Read the model definition and answer for the solid it produces. Units are mm, in the model's axes. Face numbers are marked on the shaded views. A direction names the side the tool comes from. Coordinates: 2 decimals unless noted, no trailing zeros. Write each loop counter-clockwise with the first axis right and the second up, starting at its lowest first coordinate (ties: lowest second). Pieces come first, ordered by that corner, then holes.
Item 1: Straight lines are drawn through the part: probe 1 along Z at (x, y) = (6.35, 2.2); probe 2 along Y at (x, z) = (10, -15) (3 decimals); probe 3 along Y at (x, z) = (10.25, -9.25). For each, find the intervals that lie inside material, in ascending order.
Item 2: Section C-C (z = -3.75) is taken. Give the vertices of the cut face in (x, y) (3 decimals), then the cut area to 3 significant figures.
Item 3: Each of these flat-tipped pins is pushed along its axis until it touches: P1, Ø6, axis at x = 7.5, y = 17, coming from the +Z side (3 decimals); P2, Ø6, axis at x = 6.35, z = -7.94, coming from the +Y side; P3, Ø5, axis at x = 10.5, z = -12, coming from the +Y side (3 decimals). Where does it stop, or does it pass through?
Item 4: A tool of negligible diameter and unlimited length cuts with its end or side. For the marked faces 1 and 2, from which of +Z, -Z, +X, -X, +Y, -Y can it reach the whole face along a straight path? Write none if from no direction.
Item 5: Section B-B (y = 2.75) is taken. Give the vertices of the cut face in (x, z), then the cut area to 3 significant figures.
Item 6: Section D-D (y = 12.25) is taken. Give the vertices of the cut face in (x, z) (3 decimals).
Item 7: Determine the mould class of the marked faces 3, 4, 5 and 6 for opening direction X: released by +X, released by -X, zero draft, split by the parting line, or undercut.
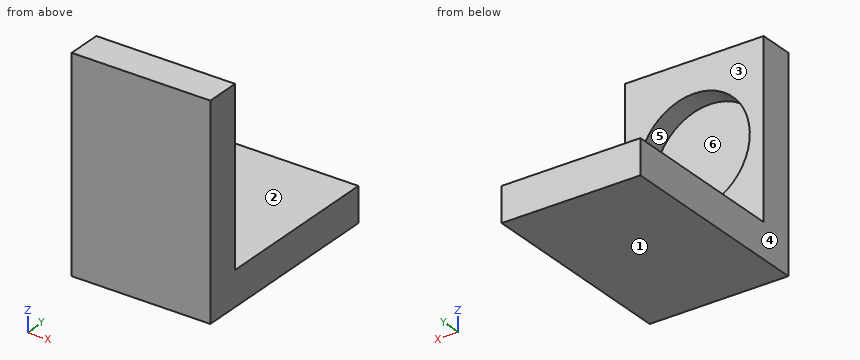
Autodesk Inventor part; units mm, degrees
ref_plane "YZ Plane" through (0, 0, 0) normal (1, 0, 0) x (0, 1, 0)
ref_plane "XZ Plane" through (0, 0, 0) normal (0, 1, 0) x (-1, 0, 0)
ref_plane "XY Plane" through (0, 0, 0) normal (0, 0, 1) x (1, 0, 0)
sketch "Sketch1" plane through (0, 0, 0) normal (1, 0, 0) x (0, 1, 0)
  line L0 (0, 0) -> (0, -19.05)
  line L1 (0, -19.05) -> (19.05, -19.05)
  line L2 (19.05, -19.05) -> (19.05, -15.875)
  line L3 (19.05, -15.875) -> (3.175, -15.875)
  line L4 (3.175, -15.875) -> (3.175, 0)
  line L5 (3.175, 0) -> (0, 0)
  dimension "d0" = 3.175
  dimension "d1" = 19.05
  dimension "d4" = 3.175
  dimension "d5" = 19.05
extrude "Extrusion1" add sketch "Sketch1" along normal blind 12.7
sketch "Sketch3" plane through (0, 3.175, 0) normal (0, 1, 0) x (1, 0, 0)
  line L0 (0, 15.875) -> (0, 0)
  line L1 (0, 0) -> (12.7, 0)
  line L2 (12.7, 15.875) -> (12.7, 0)
  line L3 (0, 15.875) -> (12.7, 15.875)
  point P0 (0, 0)
  point P1 (6.35, 7.9375)
hole "Hole2" at (6.35, 3.175, -7.9375) direction (0, -1, 0) diameter 10.16 depth 2.032
equation "\"d4\" = d0"
equation "\"d5\" = d1"
properties part number "spring tab for on arm"
Established:
1. probe 1: z = -19.05 to -13.02, -2.86 to 0
1. probe 2: y = 0 to 3.175
1. probe 3: y = 0 to 1.14
2. outline: (0, 0) - (12.7, 0) - (12.7, 3.175) - (9.226, 3.175) - (9.226, 1.143) - (3.474, 1.143) - (3.474, 3.175) - (0, 3.175) - close
2. area: 28.6 mm2
3. P1: stops at z = -15.875
3. P2: stops at y = 1.14
3. P3: stops at y = 3.175
4. face 1: -Z, +X, -X, +Y, -Y
4. face 2: +Z, +X, -X, +Y
5. outline: (0, -19.05) - (12.7, -19.05) - (12.7, 0) - (0, 0) - close; hole circle Ø10.16 at (6.35, -7.94)
5. area: 161 mm2
6. outline: (0, -19.05) - (12.7, -19.05) - (12.7, -15.875) - (0, -15.875) - close
7. face 3: zero draft
7. face 4: released by -X
7. face 5: undercut
7. face 6: undercut
